Part model, mm, in its own coordinate system. A direction names the side the tool comes from. Round coordinates to 2 decimals unless told otherwise and drop trailing zeros. Loops run counter-clockwise (first coordinate to the right, second up) from the corner with the lowest first, then second, coordinate; pieces in that order, holes last. Notation, with made-up numbers: (-36, 47) - (-28, 47) arc R14 ccw to (-28, 71) - close; hole circle Ø7 at (-38.5, 51.25). An arc over 180 degrees is marked (long way). Write each question's results on one line, items separated by ' | '. Start each with the question number.
(1) Cut at A-A, the plane z = 795.5. List the corners of the cut face in (x, y), then the cut area to 3 significant figures.
(2) Tool access for faces 1 (the face through (-1, 25, 14)), 2 (the face through (-39, 0, 1025)): list every direction of +Z, -Z, +X, -X, +Y, -Y with a clear straight run to the whole face (end or side of a thin tool).
(3) Flat gauge pins, fed straight in: P1, Ø10, axis at y = -4, z = 142, coming from the -X side; P2, Ø1.8, axis at y = -24, z = -491, coming from the -X side; P3, Ø22, axis at y = -3, z = -116, coming from the +X side; P4, Ø12, axis at x = -39, z = 511.5, coming from the +Y side. Where does each tip first touch, or does it go through?
(4) Drill centre lines: L1, parallel to Y at x = 50, z = 1029.5; L2, parallel to Z at x = -33.5, y = 9.5; L3, parallel to Y at x = 33, z = -932. Where is each one in solid material? Low to high.
(5) Mould opens along Z. For faces 3 (the face through (1, 0, 1035)), 4 (the face through (40, 0, -1025)), 5 (the face through (40, 0, 1025)), 6 (the face through (1, -25, 14)) say: released by +Z, released by -Z, zero draft, split by the parting line, or undercut.
from build123d import *

# Parameters (mm, degrees)
MEMBER_5_1_DEPTH    = 2050
MEMBER_5_2_DEPTH    = 2050
EXTRUDE_1_DEPTH     = 10
SKETCH_14_R         = 7
CUT_EXTRUDE_1_DEPTH = 10


with BuildPart() as part:
    # Sketch 11 → Member 5_1 (new body)
    with BuildSketch(Plane(origin=(0, 0, 1025), x_dir=(1, 0, 0), z_dir=(0, 0, -1))):
        with BuildLine():
            Line((0, -25), (37, -25))
            Line((37, -25), (37, -22.792319516))
            ThreePointArc((37, -22.792319516), (36.095071711, -20.443787461), (33.848226964, -19.309685745))
            Line((33.848226964, -19.309685745), (10.803546073, -17.005458605))
            ThreePointArc((10.803546073, -17.005458605), (6.309856578, -14.737255173), (4.5, -10.040191063))
            Line((4.5, -10.040191063), (4.5, 10.040191063))
            ThreePointArc((4.5, 10.040191063), (6.309856578, 14.737255173), (10.803546073, 17.005458605))
            Line((10.803546073, 17.005458605), (33.848226964, 19.309685745))
            ThreePointArc((33.848226964, 19.309685745), (36.095071711, 20.443787461), (37, 22.792319516))
            Line((37, 22.792319516), (37, 25))
            Line((37, 25), (0, 25))
            Line((0, 25), (0, -25))
        make_face()
    extrude(amount=MEMBER_5_1_DEPTH)



with BuildPart() as body_2:
    # Sketch 12 → Member 5_2 (new body)
    with BuildSketch(Plane(origin=(0, 0, 1025), x_dir=(-1, 0, 0), z_dir=(0, 0, -1))):
        with BuildLine():
            Line((0, -25), (37, -25))
            Line((37, -25), (37, -22.792319516))
            ThreePointArc((37, -22.792319516), (36.095071711, -20.443787461), (33.848226964, -19.309685745))
            Line((33.848226964, -19.309685745), (10.803546073, -17.005458605))
            ThreePointArc((10.803546073, -17.005458605), (6.309856578, -14.737255173), (4.5, -10.040191063))
            Line((4.5, -10.040191063), (4.5, 10.040191063))
            ThreePointArc((4.5, 10.040191063), (6.309856578, 14.737255173), (10.803546073, 17.005458605))
            Line((10.803546073, 17.005458605), (33.848226964, 19.309685745))
            ThreePointArc((33.848226964, 19.309685745), (36.095071711, 20.443787461), (37, 22.792319516))
            Line((37, 22.792319516), (37, 25))
            Line((37, 25), (0, 25))
            Line((0, 25), (0, -25))
        make_face()
    extrude(amount=MEMBER_5_2_DEPTH)


with BuildPart() as part_1:
    add(part.part)

    add(body_2.part)  # Extrude 1 merges body 2
    # Sketch 13 → Extrude 1 (add)
    with BuildSketch(Plane.XY.offset(1025)):
        with BuildLine():
            Line((50, -25), (0, -25))
            Line((0, -25), (-50, -25))
            ThreePointArc((-50, -25), (-75, 0), (-50, 25))
            Line((-50, 25), (0, 25))
            Line((0, 25), (50, 25))
            ThreePointArc((50, 25), (75, 0), (50, -25))
        make_face()
    extrude_1 = extrude(amount=EXTRUDE_1_DEPTH)

    # Sketch 14 → Cut-Extrude 1 (cut)
    with BuildSketch(Plane.XY.offset(1035)):
        with Locations((-50, 0)):
            Circle(SKETCH_14_R)
        with Locations((50, 0)):
            Circle(SKETCH_14_R)
    cut_extrude_1 = extrude(amount=-CUT_EXTRUDE_1_DEPTH, mode=Mode.SUBTRACT)

    # Mirror 4: Extrude 1, Cut-Extrude 1 across plane
    add(extrude_1.mirror(Plane.XY))
    add(cut_extrude_1.mirror(Plane.XY), mode=Mode.SUBTRACT)


solid = part_1.part
A:
1) outline: (-37, -25) - (37, -25) - (37, -22.79) arc R3.5 ccw to (33.85, -19.31) - (10.8, -17.01) arc R7 cw to (4.5, -10.04) - (4.5, 10.04) arc R7 cw to (10.8, 17.01) - (33.85, 19.31) arc R3.5 ccw to (37, 22.79) - (37, 25) - (-37, 25) - (-37, 22.79) arc R3.5 ccw to (-33.85, 19.31) - (-10.8, 17.01) arc R7 cw to (-4.5, 10.04) - (-4.5, -10.04) arc R7 cw to (-10.8, -17.01) - (-33.85, -19.31) arc R3.5 ccw to (-37, -22.79) - close | area: 1,380 mm2
2) face 1: +Z, -Z, +X, -X, +Y | face 2: -X
3) P1: x = -4.5 | P2: x = -37 | P3: x = 5.73 | P4: y = 25
4) L1: -25 to -7, 7 to 25 | L2: -1035 to -1025, 1025 to 1035 | L3: -25 to -19.22, 19.22 to 25
5) face 3: released by +Z | face 4: undercut | face 5: undercut | face 6: zero draft
